Verification items for the finished model (mm, model axes). Face numbers are marked on the shaded views. A direction names the side the tool comes from. Coordinates: 2 decimals unless noted, no trailing zeros. Order: outer loops, then holes, each group sorted by start corner. A loop starts at its lowest first (then second) coordinate and runs counter-clockwise, first axis right, second up.
Q1. Set-up check for the marked faces 4 and 5: record each of +Z, -Z, +X, -X, +Y, -Y from which the full face is reachable in a straight line by a thin tool's end or side.
Q2. Draft check along Z on the marked faces 1, 2 and 3. Enter one of: pulls with the +Z half, pulls with the -Z half, needs draft (parallel to the pull), parting line crosses it, or undercut.
Q3. Thickness scan on line 1 (X direction, y = 3.85, z = -3); line 2 (X direction, y = 1.7, z = 3.5). Record the ranges inside material, lowest first.
Q4. Cross-section at A-A, the plane x = -3. Count the separate pieces of the cut face and the enclosed holes in it, and give its area (3 significant figures).
Q5. Cross-section at B-B, the plane z = -5.5. Record the boundary of the cut face in (x, y), and give its area (3 significant figures).
Q6. Cross-section at C-C, the plane z = 7. Record the boundary of the cut face in (x, y).
Autodesk Inventor part; units mm, degrees
ref_plane "YZ Plane" through (0, 0, 0) normal (1, 0, 0) x (0, 1, 0)
ref_plane "XZ Plane" through (0, 0, 0) normal (0, 1, 0) x (-1, 0, 0)
ref_plane "XY Plane" through (0, 0, 0) normal (0, 0, 1) x (1, 0, 0)
sketch "スケッチ1" plane through (0, 0, 0) normal (0, 1, 0) x (-1, 0, 0)
  point P0 (0, 0)
  point P1 (4.6985, 0)
  point P2 (6.4922, 1.415)
sketch "スケッチ2" plane through (0, 0, 0) normal (0, 1, 0) x (-1, 0, 0)
  line L0 (3.75, 15.708) -> (-3.75, 15.708)
  line L1 (-3.75, 15.708) -> (-3.75, -15.708)
  line L2 (-3.75, -15.708) -> (3.75, -15.708)
  line L3 (3.75, -15.708) -> (3.75, 15.708)
  line L4 (3.75, 15.708) -> (-3.75, -15.708)
  line L5 (3.75, -15.708) -> (-3.75, 15.708)
  point P0 (0, 0)
  point P1 (0.0816, -5.789)
  point P2 (0, 0)
  dimension "d2" = 7.5
  dimension "d3" = 31.4159
extrude "押し出し1" add sketch "スケッチ2" along normal blind 5
ref_plane "作業平面1" through (0, 5, 0) normal (0, 1, 0) x (1, 0, 0)
sketch "スケッチ3" plane through (0, 5, 0) normal (0, 1, 0) x (1, 0, 0)
  line L0 (-3.75, 15.708) -> (-3.75, -15.708)
  line L1 (-3.75, -12.5664) -> (3.75, -12.5664)
  line L2 (3.75, -15.708) -> (3.75, 15.708)
  line L3 (-3.75, -15.708) -> (3.75, -15.708)
  line L4 (-3.75, -14.1372) -> (3.75, -14.1372)
  line L5 (-2.75, -15.708) -> (-2.75, -12.5664)
  line L6 (-1.5, -15.708) -> (-1.5, -12.5664)
  line L7 (-3.75, -14.5586) -> (-1.5, -15.3775)
  line L8 (-3.75, -14.5586) -> (-1.3556, -14.5586) construction
  line L9 (-3.75, -13.7157) -> (-1.5, -12.8968)
  line L10 (-3.75, -13.7157) -> (-1.3556, -13.7157) construction
  point P0 (0, 0)
  point P1 (-2.75, -14.9226)
  point P2 (-2.75, -13.3518)
  dimension "d8" = 1.5708
  dimension "d9" = 1.5708
  dimension "d10" = 1
  dimension "d11" = 1.25
  dimension "d12" = 0.7854
  dimension "d13" = 0.7854
  dimension "d14" = 20
  dimension "d15" = 20
extrude "押し出し2" cut sketch "スケッチ3" against normal blind 5 contours L1 L5 L9 L0 | L1 L6 L9 L5 | L7 L5 L3 L0 | L7 L6 L3 L5
fillet "フィレット1" radius 0.3 2 edges at (-1.5, 2.5, 12.8968) (-1.5, 2.5, 15.3775)
chamfer "面取り1" distance 0.1 angle 45 2 edges at (-3.75, 2.5, 14.5586) (-3.75, 2.5, 13.7157)
pattern_linear "矩形状パターン1" count 10 spacing 3.1416 along (0, 0, -1) of "押し出し2", "面取り1", "フィレット1"
equation "\"module\" = 1"
properties part number "lack1"
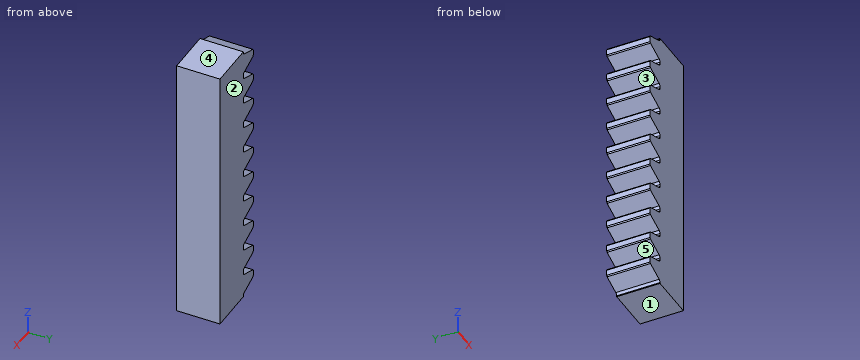
Check values:
1. face 4: +Z, +X, -X, +Y, -Y
1. face 5: -X, +Y, -Y
2. face 1: pulls with the -Z half
2. face 2: needs draft
2. face 3: undercut
3. line 1: x = -1.5 to 3.75
3. line 2: x = -1.62 to 3.75
4. separate pieces: 10
4. enclosed holes: 0
4. area: 69.4 mm2
5. outline: (-2.74, 0) - (3.75, 0) - (3.75, 5) - (-2.74, 5) - close
5. area: 32.5 mm2
6. outline: (-2.56, 0) - (3.75, 0) - (3.75, 5) - (-2.56, 5) - close
